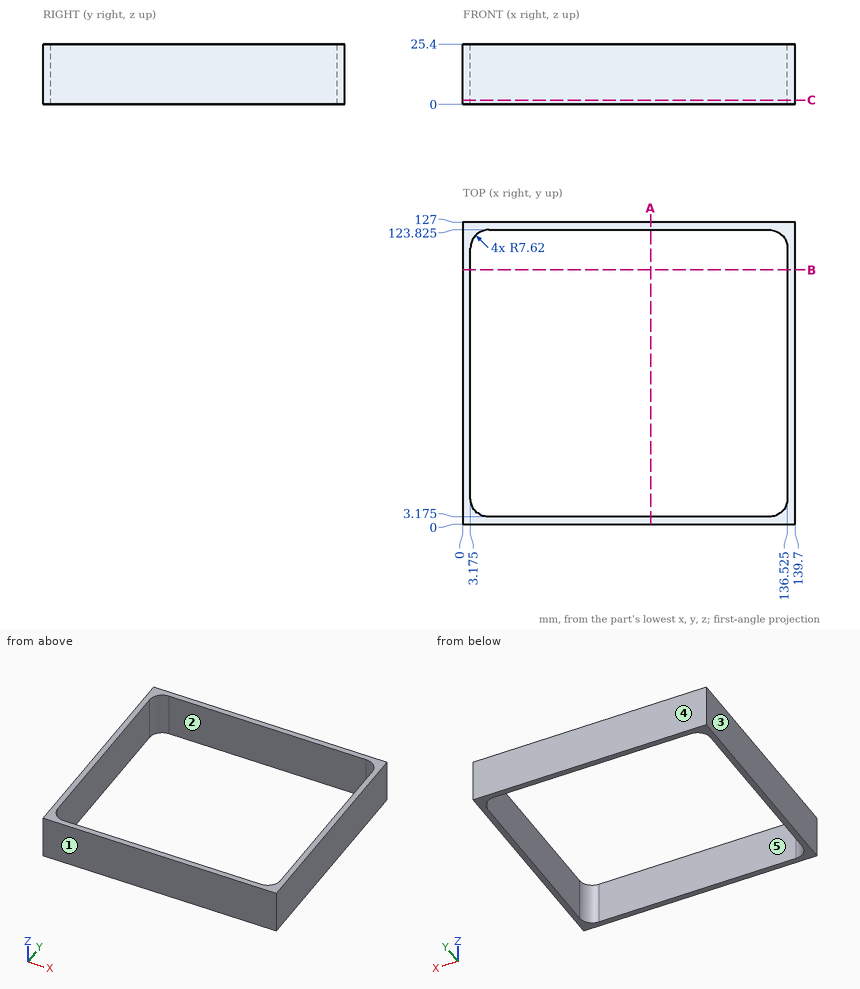
Could you check a few things on this drawing? It's one solid part, dimensions in mm from its lowest x, y, z. A direction names the side the tool comes from. Round coordinates to 2 decimals unless told otherwise and drop trailing zeros. Order: outer loops, then holes, each group sorted by start corner. A loop starts at its lowest first (then second) coordinate and runs counter-clockwise, first axis right, second up.
Q1. Thinking about a two-plate mould opening in X: for the marked faces 1, 2 and 3, which applies, released by +X, released by -X, zero draft, split by the parting line, or undercut?
Geometry says:
face 1: zero draft
face 2: undercut
face 3: released by -X
Q2. Imagine slicing it at B-B, the plane y = 107. List the corners of the cut face in (x, z) for me (3 decimals).
Geometry says:
outline: (0, 0) - (3.175, 0) - (3.175, 25.4) - (0, 25.4) - close; (136.525, 0) - (139.7, 0) - (139.7, 25.4) - (136.525, 25.4) - close
Q3. I'm going to push a flat-ended pin straight in: P1, Ø12.5, axis at y = 85.5, z = 9, coming from the -X side. Where does the tip first touch, or does it pass through?
Geometry says:
P1: stops at x = 0
Q4. Which directions (+Z, -Z, +X, -X, +Y, -Y) give clear straight access to the entire face, cutting with the end or side of a thin tool? Please do the marked faces 4 and 5.
Geometry says:
face 4: +Z, -Z, +X, -X, +Y
face 5: +Z, -Z
Q5. Imagine slicing it at A-A, the plane x = 79. List the corners of the cut face in (y, z) for me (3 decimals).
Geometry says:
outline: (0, 0) - (3.175, 0) - (3.175, 25.4) - (0, 25.4) - close; (123.825, 0) - (127, 0) - (127, 25.4) - (123.825, 25.4) - close
Q6. Imagine slicing it at C-C, the plane z = 1.75. List the corners of the cut face in (x, y) for me (3 decimals).
Geometry says:
outline: (0, 0) - (139.7, 0) - (139.7, 127) - (0, 127) - close; hole (3.175, 10.795) arc R7.62 ccw to (10.795, 3.175) - (128.905, 3.175) arc R7.62 ccw to (136.525, 10.795) - (136.525, 116.205) arc R7.62 ccw to (128.905, 123.825) - (10.795, 123.825) arc R7.62 ccw to (3.175, 116.205) - close
Q7. Please list where these lines run through material, in increasing order: probe 1 along Y at (x, z) = (45.5, 5.5) (3 decimals); probe 2 along X at (y, z) = (50, 2.5) (3 decimals); probe 3 along X at (y, z) = (121, 6.25).
Geometry says:
probe 1: y = 0 to 3.175, 123.825 to 127
probe 2: x = 0 to 3.175, 136.525 to 139.7
probe 3: x = 0 to 4.87, 134.83 to 139.7
